Geometry check sheet. Reference: the model listing, model coordinates, mm. A direction names the side the tool comes from. Coordinates: 2 decimals unless noted, no trailing zeros. Loops run counter-clockwise (first coordinate to the right, second up) from the corner with the lowest first, then second, coordinate; pieces in that order, holes last.
from build123d import *

# Parameters (mm, degrees)
SCHIZZO1_W                   = 150
SCHIZZO1_H                   = 60
ESTRUSIONE_ESTRUSIONE1_DEPTH = 4
SCHIZZO5_R                   = 1.75
ESTRUSIONE_ESTRUSIONE3_DEPTH = 4
SPECCHIA6_COPY_1_SKETCH_R    = 1.75
SPECCHIA6_COPY_1_DEPTH       = 4
RACCORDO2_R                  = 10
ESTRUSIONE_ESTRUSIONE4_DEPTH = 4
SPECCHIA8_COPY_1_DEPTH       = 4


with BuildPart() as part:
    # Schizzo1 → Estrusione-Estrusione1 (new body)
    with BuildSketch(Plane.XY):
        Rectangle(SCHIZZO1_W, SCHIZZO1_H)
    extrude(amount=ESTRUSIONE_ESTRUSIONE1_DEPTH)

    # Schizzo5 → Estrusione-Estrusione3 (add)
    with BuildSketch(Plane(origin=(0, 0, 0), x_dir=(-1, 0, 0), z_dir=(0, 0, -1))):
        with BuildLine():
            Line((-75, 30), (-68, 30))
            Line((-68, 30), (-68, 33))
            ThreePointArc((-68, 33), (-71.5, 36.5), (-75, 33))
            Line((-75, 33), (-75, 30))
        make_face()
        with Locations((-71.5, 33)):
            Circle(SCHIZZO5_R, mode=Mode.SUBTRACT)
    estrusione_estrusione3 = extrude(amount=-ESTRUSIONE_ESTRUSIONE3_DEPTH)

    # Specchia5: Estrusione-Estrusione3 across plane
    add(estrusione_estrusione3.mirror(Plane(origin=(0, 0, 0), x_dir=(0, 0, 1), z_dir=(1, 0, 0))))

    # Specchia6: Estrusione-Estrusione3 across plane
    add(estrusione_estrusione3.mirror(Plane.ZX))

    # Specchia6 copy 1 sketch → Specchia6 copy 1 (add)
    with BuildSketch(Plane(origin=(0, 0, 0), x_dir=(1, 0, 0), z_dir=(0, 0, -1))):
        with BuildLine():
            Line((-75, 30), (-68, 30))
            Line((-68, 30), (-68, 33))
            ThreePointArc((-68, 33), (-71.5, 36.5), (-75, 33))
            Line((-75, 33), (-75, 30))
        make_face()
        with Locations((-71.5, 33)):
            Circle(SPECCHIA6_COPY_1_SKETCH_R, mode=Mode.SUBTRACT)
    extrude(amount=-SPECCHIA6_COPY_1_DEPTH)

    # Raccordo2
    raccordo2_edges = [part.edges().sort_by_distance(p)[0] for p in [
        (68, -30, 2),
        (-68, -30, 2),
        (68, 30, 2),
        (-68, 30, 2),
    ]]
    fillet(raccordo2_edges, radius=RACCORDO2_R)

    # Schizzo6 → Estrusione-Estrusione4 (add)
    with BuildSketch(Plane(origin=(75, 0, 0), x_dir=(0, 0, -1), z_dir=(1, 0, 0))):
        Polygon((0, -26), (3, -25.5), (3, -18.5), (0, -18), align=None)
    estrusione_estrusione4 = extrude(amount=-ESTRUSIONE_ESTRUSIONE4_DEPTH)

    # Specchia7: Estrusione-Estrusione4 across plane
    add(estrusione_estrusione4.mirror(Plane(origin=(0, 0, 0), x_dir=(0, 0, 1), z_dir=(1, 0, 0))))

    # Specchia8: Estrusione-Estrusione4 across plane
    add(estrusione_estrusione4.mirror(Plane.ZX))

    # Specchia8 copy 1 sketch → Specchia8 copy 1 (add)
    with BuildSketch(Plane(origin=(-75, 0, 0), x_dir=(0, 0, -1), z_dir=(-1, 0, 0))):
        Polygon((0, -26), (3, -25.5), (3, -18.5), (0, -18), align=None)
    extrude(amount=-SPECCHIA8_COPY_1_DEPTH)


solid = part.part
1) Section check B-B on x = 37. Record the cut outline in (y, z).
Data:
outline: (-30, 0) - (30, 0) - (30, 4) - (-30, 4) - close
2) Depth check by flat-ended pin: pin 1 (3 mm diameter, centred on x = -9, z = 1.5, fed in from -Y); pin 2 (8 mm diameter, centred on x = 52.5, y = 25, fed in from -Z); pin 3 (2 mm diameter, centred on x = 18.5, z = 2, fed in from +Y). Enter the tip coordinate at first touch or a pass-through.
Data:
pin 1: stops at y = -30
pin 2: stops at z = 0
pin 3: stops at y = 30
3) Access from +Z, -Z, +X, -X, +Y, -Y to the whole of each face (thin tool, end or side, straight path). Record for faces 5 (the flat face through (71, 22, -1)), 6 (the flat face through (-73.028, -18.254, -1.521)), 7 (the flat face through (-1, 30, 2)).
Data:
face 5: -Z, +Y, -Y
face 6: -Z, +X, -X
face 7: +Z, -Z, +Y
4) Material ranges on probe 1 along Y at (x, z) = (-71.5, 2.3); probe 2 along X at (y, z) = (-33, 1.6); probe 3 along Y at (x, z) = (-52, 2.5), recorded low to high.
Data:
probe 1: y = -36.5 to -34.75, -31.25 to 31.25, 34.75 to 36.5
probe 2: x = -75 to -73.25, -69.75 to -67.1, 67.1 to 69.75, 73.25 to 75
probe 3: y = -30 to 30
5) Section check A-A on z = 2.25. Count the separate pieces of the cut face and the enclosed holes in it, and give its area (3 significant figures).
Data:
separate pieces: 1
enclosed holes: 4
area: 9,160 mm2
6) Section check C-C on y = 8. Record the cut outline in (x, z).
Data:
outline: (-75, 0) - (75, 0) - (75, 4) - (-75, 4) - close
7) Mould release check, pull along Y, two halves, no side actions. Record for faces 1 (the flat face through (-75, 0, 1)), 2 (the flat face through (-73.028, 18.254, -1.521)), 3 (the cylindrical face through (-72.381, -36.387, 1.972)), 4 (the flat face through (73.028, 25.754, -1.479)): +Y half, -Y half, draft (parallel to the pull), parting line (faces both ways), or undercut.
Data:
face 1: draft
face 2: undercut
face 3: -Y half
face 4: +Y half
